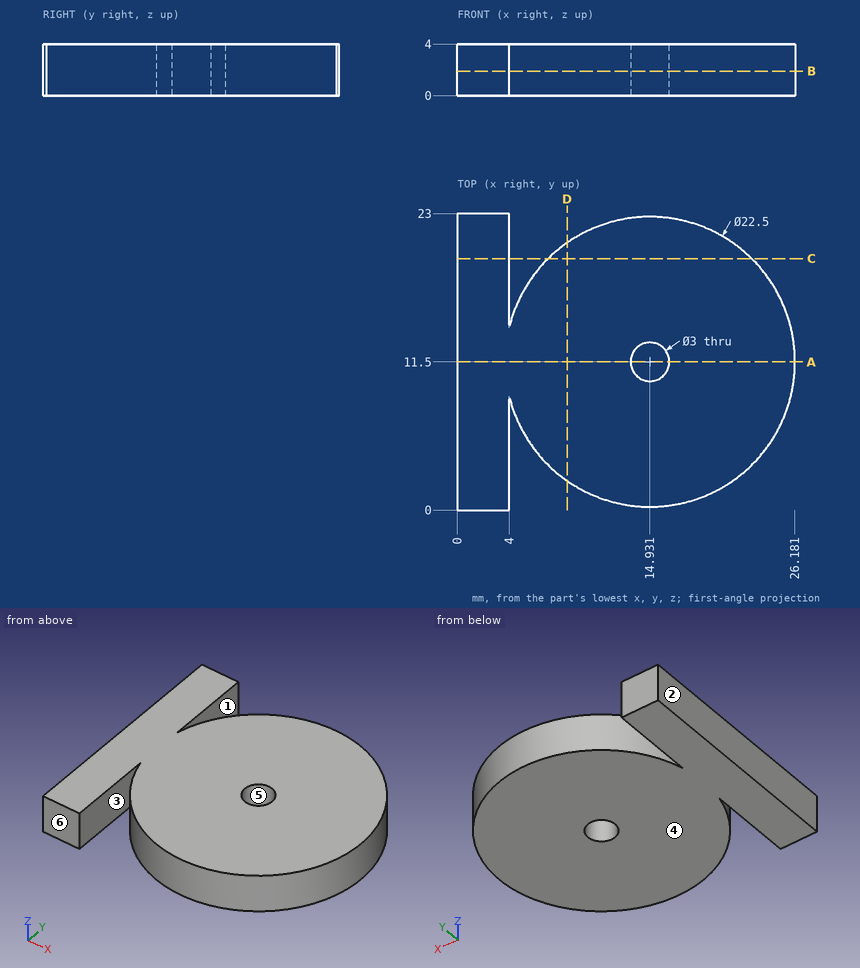
Drawing for the job (mm, zero at the part's lowest x, y, z). A direction names the side the tool comes from. Round coordinates to 2 decimals unless told otherwise and drop trailing zeros. Loops run counter-clockwise (first coordinate to the right, second up) from the corner with the lowest first, then second, coordinate; pieces in that order, holes last. Notation, with made-up numbers: (89, -26) -> (122, -26) arc R22 ccw to (122, 4) -> close; hole circle Ø7 at (84, -16). An arc over 180 degrees is marked (long way). Answer in a Markdown table with one row per item.
Item 1: Drill centre lines: L1, parallel to X at y = 16.75, z = 1.4; L2, parallel to X at y = 15.75, z = 2.75 (1 decimal); L3, parallel to Y at x = 12.5, z = 2.6 (1 decimal). Where is each one in solid material? Low to high. Write a range as [from, to].
Answers below:
| item | result |
|---|---|
| L1 | x = [0, 4], [4.98, 24.88] |
| L2 | x = [0, 4], [4.5, 25.3] |
| L3 | y = [0.5, 22.5] |
Item 2: Saw through at B-B (z = 1.9). Write the cut outline in (x, y).
Answers below:
| item | result |
|---|---|
| outline | (0, 0) -> (4, 0) -> (4, 8.84) arc R11.25 ccw (long way) to (4, 14.16) -> (4, 23) -> (0, 23) -> close; hole circle Ø3 at (14.93, 11.5) |
Item 3: Pin check, flat tip, straight feed: pin 1 (2 mm diameter, centred on y = 3, z = 1, fed in from +X). Stop position of the tip, or through.
Answers below:
| item | result |
|---|---|
| pin 1 | stops at x = 23.32 |
Item 4: Which spindle directions (+Z, -Z, +X, -X, +Y, -Y) get a long thin tool onto all of the face, cutting with end or side? Do the marked faces 1, 2 and 3. Say none if no direction does.
Answers below:
| item | result |
|---|---|
| face 1 | +Z, -Z, +Y |
| face 2 | +Z, -Z, -X, +Y, -Y |
| face 3 | +Z, -Z, -Y |
Item 5: Saw through at A-A (y = 11.5). Write the cut outline in (x, z).
Answers below:
| item | result |
|---|---|
| outline | (0, 0) -> (13.43, 0) -> (13.43, 4) -> (0, 4) -> close; (16.43, 0) -> (26.18, 0) -> (26.18, 4) -> (16.43, 4) -> close |
Item 6: Saw through at D-D (x = 8.5). Write the cut outline in (y, z).
Answers below:
| item | result |
|---|---|
| outline | (2.27, 0) -> (20.73, 0) -> (20.73, 4) -> (2.27, 4) -> close |
Item 7: Saw through at C-C (y = 19.5). Write the cut outline in (x, z).
Answers below:
| item | result |
|---|---|
| outline | (0, 0) -> (4, 0) -> (4, 4) -> (0, 4) -> close; (7.02, 0) -> (22.84, 0) -> (22.84, 4) -> (7.02, 4) -> close |
Item 8: Mould opens along Y. For the marked faces 4, 5 and 6 say: +Y half, -Y half, draft (parallel to the pull), parting line (faces both ways), or undercut.
Answers below:
| item | result |
|---|---|
| face 4 | draft |
| face 5 | undercut |
| face 6 | -Y half |
